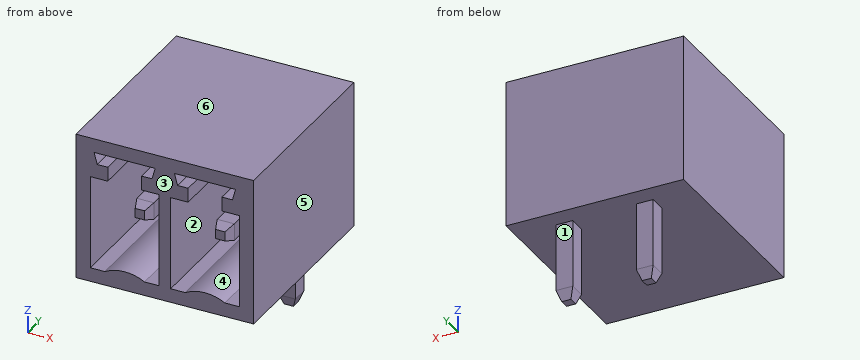
from build123d import *
from OCP.BRepFilletAPI import BRepFilletAPI_MakeChamfer

# Parameters (mm, degrees)
SKETCH1_W                    = 8.42
SKETCH1_H                    = 9.2
BOSS_EXTRUDE1_DEPTH          = 7
CUT_EXTRUDE1_DEPTH           = 7
LPATTERN1_COUNT              = 2
LPATTERN1_PITCH              = 3.81
SKETCH3_R                    = 0.875
BOSS_EXTRUDE2_DEPTH          = 1.15
CHAMFER1_SIZE                = 0.5
CHAMFER1_SIZE2               = 0.056791013
SKETCH4_W                    = 0.81
SKETCH4_H                    = 0.81
BOSS_EXTRUDE3_DEPTH          = 4.45
CHAMFER2_SIZE                = 0.5
CHAMFER2_SIZE2               = 0.181985117
LPATTERN3_COUNT              = 2
LPATTERN3_PITCH              = 3.81
CHAMFER1_OF_LPATTERN3_SIZE2  = 0.056791013
CHAMFER1_OF_LPATTERN3_SIZE   = 0.5
LPATTERN4_COUNT              = 2
LPATTERN4_PITCH              = 3.81
CHAMFER2_OF_LPATTERN4_SIZE   = 0.5
CHAMFER2_OF_LPATTERN4_SIZE2  = 0.181985117
BOSS_EXTRUDE4_START          = -3.4
SKETCH5_W                    = 0.8
SKETCH5_H                    = 0.8
BOSS_EXTRUDE4_DEPTH          = 7.1
CHAMFER3_SIZE                = 0.5
CHAMFER3_SIZE2               = 0.181985117
LPATTERN12_COUNT             = 2
LPATTERN12_PITCH             = 3.81
CHAMFER3_OF_LPATTERN12_SIZE  = 0.5
CHAMFER3_OF_LPATTERN12_SIZE2 = 0.181985117


with BuildPart() as part:
    # Sketch1 → Boss-Extrude1 (new body)
    with BuildSketch(Plane.XY):
        Rectangle(SKETCH1_W, SKETCH1_H)
    extrude(amount=BOSS_EXTRUDE1_DEPTH)

    # Sketch2 → Cut-Extrude1 (cut)
    with BuildSketch(Plane.XZ.offset(4.6)):
        with BuildLine():
            Line((-3.535, 5.11), (-2.705, 5.11))
            Line((-2.705, 5.11), (-2.705, 5.79))
            Line((-2.705, 5.79), (-3.205, 5.79))
            Line((-3.205, 5.79), (-3.353813394, 6.34))
            Line((-3.353813394, 6.34), (-0.456186606, 6.34))
            Line((-0.456186606, 6.34), (-0.605, 5.79))
            Line((-0.605, 5.79), (-1.105, 5.79))
            Line((-1.105, 5.79), (-1.105, 5.11))
            Line((-1.105, 5.11), (-0.275, 5.11))
            Line((-0.275, 5.11), (-0.275, 0.66))
            Line((-0.275, 0.66), (-0.965, 0.66))
            ThreePointArc((-0.965, 0.66), (-1.905, 0.904), (-2.845, 0.66))
            Line((-2.845, 0.66), (-3.535, 0.66))
            Line((-3.535, 0.66), (-3.535, 5.11))
        make_face()
    cut_extrude1 = extrude(amount=-CUT_EXTRUDE1_DEPTH, mode=Mode.SUBTRACT)

    # LPattern1: Cut-Extrude1 ×2
    with Locations(*[(i * LPATTERN1_PITCH, 0, 0) for i in range(1, LPATTERN1_COUNT)]):
        add(cut_extrude1, mode=Mode.SUBTRACT)

    # Sketch3 → Boss-Extrude2 (add)
    with BuildSketch(Plane.XZ.offset(-2.4)):
        with Locations(Location((-1.905, 2.985, 0), (0, 0, 90))):
            Circle(SKETCH3_R)
    boss_extrude2 = extrude(amount=BOSS_EXTRUDE2_DEPTH)

    # Chamfer1
    chamfer1_edges = [part.edges().sort_by_distance(p)[0] for p in [
        (-1.905, 1.25, 2.11),
    ]]
    chamfer1_side = [part.faces().sort_by_distance(p)[0] for p in [
        (-1.905, 1.825, 2.11),
    ]]
    chamfer(chamfer1_edges, length=CHAMFER1_SIZE, length2=CHAMFER1_SIZE2, reference=chamfer1_side[0])

    # Sketch4 → Boss-Extrude3 (add)
    with BuildSketch(Plane.XZ.offset(-1.25)):
        with Locations((-1.905, 2.985)):
            Rectangle(SKETCH4_W, SKETCH4_H)
    boss_extrude3 = extrude(amount=BOSS_EXTRUDE3_DEPTH)

    # Chamfer2: one chamfer whose edges measure the first distance from different faces: ONE call of the kernel's chamfer builder (chamfer() names one face for all edges)
    chamfer2_edges_1 = [part.edges().sort_by_distance(p)[0] for p in [
        (-1.5, -3.2, 2.985),
    ]]
    chamfer2_side_1 = [part.faces().sort_by_distance(p)[0] for p in [
        (-1.5, -0.975, 2.985),
    ]]
    chamfer2_edges_2 = [part.edges().sort_by_distance(p)[0] for p in [
        (-1.905, -3.2, 3.39),
    ]]
    chamfer2_side_2 = [part.faces().sort_by_distance(p)[0] for p in [
        (-1.905, -0.975, 3.39),
    ]]
    chamfer2_edges_3 = [part.edges().sort_by_distance(p)[0] for p in [
        (-2.31, -3.2, 2.985),
    ]]
    chamfer2_side_3 = [part.faces().sort_by_distance(p)[0] for p in [
        (-2.31, -0.975, 2.985),
    ]]
    chamfer2_edges_4 = [part.edges().sort_by_distance(p)[0] for p in [
        (-1.905, -3.2, 2.58),
    ]]
    chamfer2_side_4 = [part.faces().sort_by_distance(p)[0] for p in [
        (-1.905, -0.975, 2.58),
    ]]
    chamfer2 = BRepFilletAPI_MakeChamfer(part.part.solid().wrapped)
    for e in chamfer2_edges_1:
        chamfer2.Add(CHAMFER2_SIZE, CHAMFER2_SIZE2, e.wrapped, chamfer2_side_1[0].wrapped)  # the first distance lies on this face
    for e in chamfer2_edges_2:
        chamfer2.Add(CHAMFER2_SIZE, CHAMFER2_SIZE2, e.wrapped, chamfer2_side_2[0].wrapped)  # the first distance lies on this face
    for e in chamfer2_edges_3:
        chamfer2.Add(CHAMFER2_SIZE, CHAMFER2_SIZE2, e.wrapped, chamfer2_side_3[0].wrapped)  # the first distance lies on this face
    for e in chamfer2_edges_4:
        chamfer2.Add(CHAMFER2_SIZE, CHAMFER2_SIZE2, e.wrapped, chamfer2_side_4[0].wrapped)  # the first distance lies on this face
    add(Compound.cast(chamfer2.Shape()), mode=Mode.REPLACE)

    # LPattern3: Boss-Extrude2 ×2
    with Locations(*[(i * LPATTERN3_PITCH, 0, 0) for i in range(1, LPATTERN3_COUNT)]):
        add(boss_extrude2)

    # Chamfer1 of LPattern3
    chamfer1_of_lpattern3_edges = [part.edges().sort_by_distance(p)[0] for p in [
        (1.905, 1.25, 2.11),
    ]]
    chamfer(chamfer1_of_lpattern3_edges, length=CHAMFER1_OF_LPATTERN3_SIZE, length2=CHAMFER1_OF_LPATTERN3_SIZE2)

    # LPattern4: Boss-Extrude3 ×2
    with Locations(*[(i * LPATTERN4_PITCH, 0, 0) for i in range(1, LPATTERN4_COUNT)]):
        add(boss_extrude3)

    # Chamfer2 of LPattern4: one chamfer whose edges measure the first distance from different faces: ONE call of the kernel's chamfer builder (chamfer() names one face for all edges)
    chamfer2_of_lpattern4_edges_1 = [part.edges().sort_by_distance(p)[0] for p in [
        (2.31, -3.2, 2.985),
    ]]
    chamfer2_of_lpattern4_side_1 = [part.faces().sort_by_distance(p)[0] for p in [
        (2.31, -0.975, 2.985),
    ]]
    chamfer2_of_lpattern4_edges_2 = [part.edges().sort_by_distance(p)[0] for p in [
        (1.905, -3.2, 3.39),
    ]]
    chamfer2_of_lpattern4_side_2 = [part.faces().sort_by_distance(p)[0] for p in [
        (1.905, -0.975, 3.39),
    ]]
    chamfer2_of_lpattern4_edges_3 = [part.edges().sort_by_distance(p)[0] for p in [
        (1.5, -3.2, 2.985),
    ]]
    chamfer2_of_lpattern4_side_3 = [part.faces().sort_by_distance(p)[0] for p in [
        (1.5, -0.975, 2.985),
    ]]
    chamfer2_of_lpattern4_edges_4 = [part.edges().sort_by_distance(p)[0] for p in [
        (1.905, -3.2, 2.58),
    ]]
    chamfer2_of_lpattern4_side_4 = [part.faces().sort_by_distance(p)[0] for p in [
        (1.905, -0.975, 2.58),
    ]]
    chamfer2_of_lpattern4 = BRepFilletAPI_MakeChamfer(part.part.solid().wrapped)
    for e in chamfer2_of_lpattern4_edges_1:
        chamfer2_of_lpattern4.Add(CHAMFER2_OF_LPATTERN4_SIZE, CHAMFER2_OF_LPATTERN4_SIZE2, e.wrapped, chamfer2_of_lpattern4_side_1[0].wrapped)  # the first distance lies on this face
    for e in chamfer2_of_lpattern4_edges_2:
        chamfer2_of_lpattern4.Add(CHAMFER2_OF_LPATTERN4_SIZE, CHAMFER2_OF_LPATTERN4_SIZE2, e.wrapped, chamfer2_of_lpattern4_side_2[0].wrapped)  # the first distance lies on this face
    for e in chamfer2_of_lpattern4_edges_3:
        chamfer2_of_lpattern4.Add(CHAMFER2_OF_LPATTERN4_SIZE, CHAMFER2_OF_LPATTERN4_SIZE2, e.wrapped, chamfer2_of_lpattern4_side_3[0].wrapped)  # the first distance lies on this face
    for e in chamfer2_of_lpattern4_edges_4:
        chamfer2_of_lpattern4.Add(CHAMFER2_OF_LPATTERN4_SIZE, CHAMFER2_OF_LPATTERN4_SIZE2, e.wrapped, chamfer2_of_lpattern4_side_4[0].wrapped)  # the first distance lies on this face
    add(Compound.cast(chamfer2_of_lpattern4.Shape()), mode=Mode.REPLACE)

    # Sketch5 → Boss-Extrude4 (add)
    with BuildSketch(Plane(origin=(0, 0, 0), x_dir=(-1, 0, 0), z_dir=(0, 0, -1)).offset(BOSS_EXTRUDE4_START)):
        with Locations((1.9, 3.3)):
            Rectangle(SKETCH5_W, SKETCH5_H)
    boss_extrude4 = extrude(amount=BOSS_EXTRUDE4_DEPTH)

    # Chamfer3: one chamfer whose edges measure the first distance from different faces: ONE call of the kernel's chamfer builder (chamfer() names one face for all edges)
    chamfer3_edges_1 = [part.edges().sort_by_distance(p)[0] for p in [
        (-1.9, 2.9, -3.7),
    ]]
    chamfer3_side_1 = [part.faces().sort_by_distance(p)[0] for p in [
        (-1.9, 2.9, -1.85),
    ]]
    chamfer3_edges_2 = [part.edges().sort_by_distance(p)[0] for p in [
        (-1.5, 3.3, -3.7),
    ]]
    chamfer3_side_2 = [part.faces().sort_by_distance(p)[0] for p in [
        (-1.5, 3.3, -1.85),
    ]]
    chamfer3_edges_3 = [part.edges().sort_by_distance(p)[0] for p in [
        (-2.3, 3.3, -3.7),
    ]]
    chamfer3_side_3 = [part.faces().sort_by_distance(p)[0] for p in [
        (-2.3, 3.3, -1.85),
    ]]
    chamfer3_edges_4 = [part.edges().sort_by_distance(p)[0] for p in [
        (-1.9, 3.7, -3.7),
    ]]
    chamfer3_side_4 = [part.faces().sort_by_distance(p)[0] for p in [
        (-1.9, 3.7, -1.85),
    ]]
    chamfer3 = BRepFilletAPI_MakeChamfer(part.part.solid().wrapped)
    for e in chamfer3_edges_1:
        chamfer3.Add(CHAMFER3_SIZE, CHAMFER3_SIZE2, e.wrapped, chamfer3_side_1[0].wrapped)  # the first distance lies on this face
    for e in chamfer3_edges_2:
        chamfer3.Add(CHAMFER3_SIZE, CHAMFER3_SIZE2, e.wrapped, chamfer3_side_2[0].wrapped)  # the first distance lies on this face
    for e in chamfer3_edges_3:
        chamfer3.Add(CHAMFER3_SIZE, CHAMFER3_SIZE2, e.wrapped, chamfer3_side_3[0].wrapped)  # the first distance lies on this face
    for e in chamfer3_edges_4:
        chamfer3.Add(CHAMFER3_SIZE, CHAMFER3_SIZE2, e.wrapped, chamfer3_side_4[0].wrapped)  # the first distance lies on this face
    add(Compound.cast(chamfer3.Shape()), mode=Mode.REPLACE)

    # LPattern12: Boss-Extrude4 ×2
    with Locations(*[(i * LPATTERN12_PITCH, 0, 0) for i in range(1, LPATTERN12_COUNT)]):
        add(boss_extrude4)

    # Chamfer3 of LPattern12: one chamfer whose edges measure the first distance from different faces: ONE call of the kernel's chamfer builder (chamfer() names one face for all edges)
    chamfer3_of_lpattern12_edges_1 = [part.edges().sort_by_distance(p)[0] for p in [
        (1.91, 2.9, -3.7),
    ]]
    chamfer3_of_lpattern12_side_1 = [part.faces().sort_by_distance(p)[0] for p in [
        (1.91, 2.9, -1.85),
    ]]
    chamfer3_of_lpattern12_edges_2 = [part.edges().sort_by_distance(p)[0] for p in [
        (2.31, 3.3, -3.7),
    ]]
    chamfer3_of_lpattern12_side_2 = [part.faces().sort_by_distance(p)[0] for p in [
        (2.31, 3.3, -1.85),
    ]]
    chamfer3_of_lpattern12_edges_3 = [part.edges().sort_by_distance(p)[0] for p in [
        (1.51, 3.3, -3.7),
    ]]
    chamfer3_of_lpattern12_side_3 = [part.faces().sort_by_distance(p)[0] for p in [
        (1.51, 3.3, -1.85),
    ]]
    chamfer3_of_lpattern12_edges_4 = [part.edges().sort_by_distance(p)[0] for p in [
        (1.91, 3.7, -3.7),
    ]]
    chamfer3_of_lpattern12_side_4 = [part.faces().sort_by_distance(p)[0] for p in [
        (1.91, 3.7, -1.85),
    ]]
    chamfer3_of_lpattern12 = BRepFilletAPI_MakeChamfer(part.part.solid().wrapped)
    for e in chamfer3_of_lpattern12_edges_1:
        chamfer3_of_lpattern12.Add(CHAMFER3_OF_LPATTERN12_SIZE, CHAMFER3_OF_LPATTERN12_SIZE2, e.wrapped, chamfer3_of_lpattern12_side_1[0].wrapped)  # the first distance lies on this face
    for e in chamfer3_of_lpattern12_edges_2:
        chamfer3_of_lpattern12.Add(CHAMFER3_OF_LPATTERN12_SIZE, CHAMFER3_OF_LPATTERN12_SIZE2, e.wrapped, chamfer3_of_lpattern12_side_2[0].wrapped)  # the first distance lies on this face
    for e in chamfer3_of_lpattern12_edges_3:
        chamfer3_of_lpattern12.Add(CHAMFER3_OF_LPATTERN12_SIZE, CHAMFER3_OF_LPATTERN12_SIZE2, e.wrapped, chamfer3_of_lpattern12_side_3[0].wrapped)  # the first distance lies on this face
    for e in chamfer3_of_lpattern12_edges_4:
        chamfer3_of_lpattern12.Add(CHAMFER3_OF_LPATTERN12_SIZE, CHAMFER3_OF_LPATTERN12_SIZE2, e.wrapped, chamfer3_of_lpattern12_side_4[0].wrapped)  # the first distance lies on this face
    add(Compound.cast(chamfer3_of_lpattern12.Shape()), mode=Mode.REPLACE)


solid = part.part
The model under review builds one solid part; all positions refer to its coordinate system, in mm. Face numbers are marked on the shaded views. A direction names the side the tool comes from. Round coordinates to 2 decimals unless told otherwise and drop trailing zeros. Order: outer loops, then holes, each group sorted by start corner. A loop starts at its lowest first (then second) coordinate and runs counter-clockwise, first axis right, second up. Notation, with made-up numbers: (2, 62) -> (40, 62) arc R15 ccw to (40, 75) -> close; hole circle Ø11 at (63.25, 46.25). An arc over 180 degrees is marked (long way). Return JSON: item names as keys, results as strings.
1. The part is to be moulded in two halves that separate along Z. For the marked faces 4, 5 and 6, say which applies: +Z half, -Z half, draft (parallel to the pull), parting line (faces both ways), or undercut.
Answer block:
{"face 4": "undercut", "face 5": "draft", "face 6": "+Z half"}
2. Insertion check: P1, Ø2, axis at x = -2.5, z = -2, coming from the +Y side; P2, Ø0.6, axis at y = 3.5, z = -1, coming from the +X side. Each pin has a flat end and moves straight along its axis. Give the tip position at first contact, or say it passes through.
Answer block:
{"P1": "stops at y = 3.7", "P2": "stops at x = 2.31"}
3. For the marked faces 1, 2 and 3, list the 3-axis set-ups (+Z, -Z, +X, -X, +Y, -Y) from which the entire face can be reached by the end or side of a thin tool; tool diameter is ignored.
Answer block:
{"face 1": "-Z, +X, -X, +Y", "face 2": "-Y", "face 3": "+Z, -Z, +X, -X, -Y"}
4. For L1, parallel to X at y = 0, z = 4.5 (3 decimals); L2, parallel to X at y = 2, z = 3 (3 decimals); L3, parallel to Z at x = -1, y = 1.5, list the stretches that pass through material, from the lowest coordinate up. Write a range as [from, to].
Answer block:
{"L1": "x = [-4.21, -3.535], [-0.275, 0.275], [3.535, 4.21]", "L2": "x = [-4.21, -3.535], [-2.78, -1.03], [-0.275, 0.275], [1.03, 2.78], [3.535, 4.21]", "L3": "z = [0, 0.68], [5.11, 5.79], [6.34, 7]"}
5. Take a section at A-A (z = -2.25). Write out the cut boundary in (x, y).
Answer block:
{"outline": "(-2.3, 2.9) -> (-1.5, 2.9) -> (-1.5, 3.7) -> (-2.3, 3.7) -> close; (1.51, 2.9) -> (2.31, 2.9) -> (2.31, 3.7) -> (1.51, 3.7) -> close"}
6. Take a section at C-C (z = 1.5). Write out the cut boundary in (x, y) (3 decimals).
Answer block:
{"outline": "(-4.21, -4.6) -> (-3.535, -4.6) -> (-3.535, 2.4) -> (-0.275, 2.4) -> (-0.275, -4.6) -> (0.275, -4.6) -> (0.275, 2.4) -> (3.535, 2.4) -> (3.535, -4.6) -> (4.21, -4.6) -> (4.21, 4.6) -> (-4.21, 4.6) -> close"}
7. Take a section at B-B (y = -4). State how many separate pieces and enclosed holes the cut face has, then the cut area to 3 significant figures.
Answer block:
{"separate pieces": "1", "enclosed holes": "2", "area": "25.3 mm²"}
